Study the drawing (mm; zero at the part's minimum x, y, z) and answer. A direction names the side the tool comes from. Give positions to 0.01 mm unless a question says otherwise; leave off trailing zeros. Order: outer loops, then holes, each group sorted by start corner. A loop starts at its lowest first (then second) coordinate and runs counter-clockwise, first axis right, second up. Notation, with made-up numbers: (-12, 11) - (9, 11) arc R25 cw to (9, 46) - close; hole circle Ø1 at (7.25, -33.5). An arc over 180 degrees is marked (long way). Return JSON: item names as keys, results as strings.
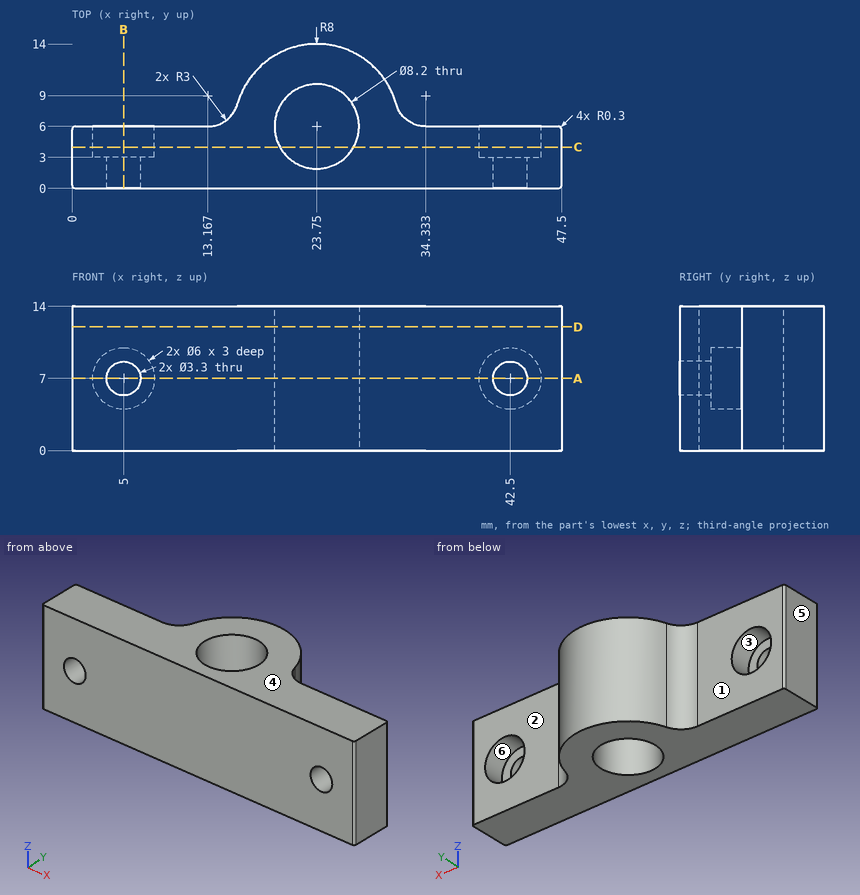
Q1. For the marked faces 1, 2 and 3, determine the directions among +Z, -Z, +X, -X, +Y, -Y from which every point of the face is accessible in a straight line to the end or side of a thin tool.
Values:
{"face 1": "+Z, -Z, -X, +Y", "face 2": "+Z, -Z, +X, +Y", "face 3": "+Y"}
Q2. Consider L1, parallel to Z at x = 42.5, y = 4.15; L2, parallel to X at y = 1.4, z = 7; L3, parallel to Z at x = 42.5, y = 1.6. Determine where each line is inside the solid, lowest interval first.
Values:
{"L1": "z = 0 to 4, 10 to 14", "L2": "x = 0 to 3.35, 6.65 to 40.85, 44.15 to 47.5", "L3": "z = 0 to 5.35, 8.65 to 14"}
Q3. A cutting plane is placed at B-B (x = 5). Write down the section's boundary in (y, z), and give its area (3 significant figures).
Values:
{"outline": "(0, 0) - (6, 0) - (6, 4) - (3, 4) - (3, 5.35) - (0, 5.35) - close; (0, 8.65) - (3, 8.65) - (3, 10) - (6, 10) - (6, 14) - (0, 14) - close", "area": "56.1 mm²"}
Q4. A cutting plane is placed at A-A (z = 7). Give the number of separate pieces and of enclosed holes in the cut face, and give its area (3 significant figures).
Values:
{"separate pieces": "3", "enclosed holes": "1", "area": "279 mm²"}
Q5. A cutting plane is placed at C-C (y = 4). Write down the section's boundary in (x, z), and give its area (3 significant figures).
Values:
{"outline": "(0, 0) - (20.17, 0) - (20.17, 14) - (0, 14) - close; (27.33, 0) - (47.5, 0) - (47.5, 14) - (27.33, 14) - close; hole circle Ø6 at (5, 7); hole circle Ø6 at (42.5, 7)", "area": "508 mm²"}
Q6. Determine the mould class of the marked faces 4, 5 and 6 for opening direction Z: released by +Z, released by -Z, zero draft, split by the parting line, or undercut.
Values:
{"face 4": "released by +Z", "face 5": "zero draft", "face 6": "undercut"}
Q7. Given pin 1 (3 mm diameter, centred on y = 8, z = 10, fed in from +X); pin 2 (1.5 mm diameter, centred on y = 10.5, z = 9.5, fed in from -X); pin 3 (6.5 mm diameter, centred on x = 7, z = 4.5, fed in from +Y), each flat-ended and moving along its own axis, determine where each tip first touches the part or whether it passes through.
Values:
{"pin 1": "stops at x = 32.67", "pin 2": "stops at x = 16.68", "pin 3": "stops at y = 6"}
Q8. A cutting plane is placed at D-D (z = 12). Write down the section's boundary in (x, y).
Values:
{"outline": "(0, 0.3) arc R0.3 ccw to (0.3, 0) - (47.2, 0) arc R0.3 ccw to (47.5, 0.3) - (47.5, 5.7) arc R0.3 ccw to (47.2, 6) - (34.33, 6) arc R3 cw to (31.45, 8.18) arc R8 ccw to (16.05, 8.18) arc R3 cw to (13.17, 6) - (0.3, 6) arc R0.3 ccw to (0, 5.7) - close; hole circle Ø8.2 at (23.75, 6)"}
